Autodesk Inventor part; units mm, degrees
ref_plane "YZ Plane" through (0, 0, 0) normal (1, 0, 0) x (0, 1, 0)
ref_plane "XZ Plane" through (0, 0, 0) normal (0, 1, 0) x (-1, 0, 0)
ref_plane "XY Plane" through (0, 0, 0) normal (0, 0, 1) x (1, 0, 0)
sketch "Szkic2" plane through (0, 0, 0) normal (1, 0, 0) x (0, 1, 0)
  line L0 (0, -2.9) -> (0, 2.9)
  line L1 (-1.5, -1.5) -> (-1.5, 1.5)
  line L2 (-1.5, -1.5) -> (0, -2.9)
  line L3 (-1.5, 1.5) -> (0, 2.9)
  line L4 (0, 0) -> (-8, 0)
  line L5 (-8, 0) -> (-8, -1.5)
  line L6 (-8, -1.5) -> (-1.5, -1.5)
  dimension "d0" = 5.8
  dimension "d2" = 3
  dimension "d3" = 1.5
  dimension "d4" = 8
  dimension "d5" = 1.5
revolve "Obrót1" add sketch "Szkic2" angle 360 about axis through (0, 0, 0) along (0, -1, 0) contours L2 L1 L4 L0 | L6 L5 L4 L1
sketch "Szkic3" plane through (0, 0, 0) normal (0, 1, 0) x (1, 0, 0)
  line L0 (-1.1673, -0.633) -> (-1.1318, 0.6945)
  line L1 (-1.1318, 0.6945) -> (0.0355, 1.3274)
  line L2 (0.0355, 1.3274) -> (1.1673, 0.633)
  line L3 (1.1673, 0.633) -> (1.1318, -0.6945)
  line L4 (1.1318, -0.6945) -> (-0.0355, -1.3274)
  line L5 (-0.0355, -1.3274) -> (-1.1673, -0.633)
  point P0 (0, 0)
  point P1 (0, 0)
  dimension "d7" = 2.3
extrude "Wyciągnięcie proste1" cut sketch "Szkic3" against normal blind 2
fillet "Zaokrąglenie1" radius 0.5 6 edges at (-1.1496, -2, -0.0308) (-0.6014, -2, 0.9802) (-0.5482, -2, -1.011) (0.6014, -2, -0.9802) (0.5482, -2, 1.011) (1.1496, -2, 0.0308)
fillet "Zaokrąglenie2" radius 0.5 1 edges at (0, -1.5, 1.5)
fillet "Zaokrąglenie3" radius 0.1 1 edges at (0, 0, 2.9)
thread "Gwint1"
chamfer "Faza1" distance 0.5 angle 45 1 edges at (0, -8, 1.5)
properties part number "Screw M3 8mm flat head"
Build history of the part. All positions in model axes, mm. A direction names the side the tool comes from. Round coordinates to 2 decimals unless told otherwise and drop trailing zeros. Order: outer loops, then holes, each group sorted by start corner. A loop starts at its lowest first (then second) coordinate and runs counter-clockwise, first axis right, second up. Notation, with made-up numbers: (-12, 79.25) - (-1, 79.25) arc R28 cw to (-1, 105.25) - close; hole circle Ø1 at (-18, 14.5). An arc over 180 degrees is marked (long way). Use a Markdown table: item, result.
1) Saw through at A-A on y = -0.5. Write the cut outline in (x, z), and give its area (3 significant figures).
Recorded:
| item | result |
|---|---|
| outline | circle Ø4.87 at (0, 0); hole (-1.17, 0.63) - (-1.13, -0.69) - (0.04, -1.33) - (1.17, -0.63) - (1.13, 0.69) - (-0.04, 1.33) - close |
| area | 14.0 mm² |
2) Saw through at B-B on y = -6.5. Write the cut outline in (x, z).
Recorded:
| item | result |
|---|---|
| outline | circle Ø3 at (0, 0) |
3) Pull direction Z, two halves, no side cores. Call faces 1 (the face through (0.593, -0.74, -0.985)), 2 (the face through (-0.07, -4.56, 1.5)), 3 (the face through (-1, 0, -1)): pulls with the +Z half, pulls with the -Z half, needs draft (parallel to the pull), parting line crosses it, or undercut.
Recorded:
| item | result |
|---|---|
| face 1 | undercut |
| face 2 | parting line crosses it |
| face 3 | needs draft |
4) Tool access for faces 4 (the face through (-0.531, -1.857, 0.847)), 5 (the face through (0, -8, 0)): list every direction of +Z, -Z, +X, -X, +Y, -Y with a clear straight run to the whole face (end or side of a thin tool).
Recorded:
| item | result |
|---|---|
| face 4 | +Y |
| face 5 | +Z, -Z, +X, -X, -Y |
5) Flat gauge pins, fed straight in: pin 1 Ø2 at (y, z) = (-6, 0) entering from -X; pin 2 Ø2 at (x, y) = (-1.5, -3) entering from -Z. Where does each tip first touch, or does it go through?
Recorded:
| item | result |
|---|---|
| pin 1 | stops at x = -1.5 |
| pin 2 | stops at z = -1.41 |
6) Wall check: L1, parallel to X at y = -1.5, z = 0.9; L2, parallel to X at y = -4, z = -0.05; L3, parallel to Y at x = 1.6, z = -0.8. Give the ranges that are in metal, low to high.
Recorded:
| item | result |
|---|---|
| L1 | x = -1.25 to -0.73, 0.75 to 1.25 |
| L2 | x = -1.5 to 1.5 |
| L3 | y = -1.19 to 0 |
